from build123d import *

# Parameters (mm, degrees)
SKETCH1_W           = 50
SKETCH1_H           = 45
BOSS_EXTRUDE1_DEPTH = 2
FILLET1_R           = 2
SKETCH3_W           = 3
SKETCH3_H           = 10
SKETCH3_W_2         = 7.936264089
SKETCH3_H_2         = 3
SKETCH3_W_3         = 11
SKETCH3_H_3         = 1.470363465
SKETCH3_H_4         = 1.529636535
SKETCH3_W_4         = 7.991276849
SKETCH3_H_5         = 45
CUT_EXTRUDE1_DEPTH  = 2
SKETCH4_R           = 2
CUT_EXTRUDE2_DEPTH  = 10


with BuildPart() as part:
    # Sketch1 → Boss-Extrude1 (new body)
    with BuildSketch(Plane.XY):
        Polygon((-65, -32.5), (65, -32.5), (65, 32.5), (25, 32.5), (25, -12.5), (-25, -12.5), (-25, 32.5), (-65, 32.5), align=None)
        with Locations((0, 55)):
            Rectangle(SKETCH1_W, SKETCH1_H)
        with Locations((0, 10)):
            Rectangle(SKETCH1_W, SKETCH1_H)
    extrude(amount=BOSS_EXTRUDE1_DEPTH)

    # Fillet1
    fillet1_edges = [part.edges().sort_by_distance(p)[0] for p in [
        (65, 32.5, 1),
        (65, -32.5, 1),
        (-65, -32.5, 1),
        (-65, 32.5, 1),
        (-25, 32.5, 1),
        (-25, 77.5, 1),
        (25, 77.5, 1),
        (25, 32.5, 1),
    ]]
    fillet(fillet1_edges, radius=FILLET1_R)

    # Sketch3 → Cut-Extrude1 (cut)
    with BuildSketch(Plane(origin=(0, 0, 0), x_dir=(-1, 0, 0), z_dir=(0, 0, -1))):
        with Locations((6, 40.5)):
            Rectangle(SKETCH3_W, SKETCH3_H)
        with Locations((-6, 40.5)):
            Rectangle(SKETCH3_W, SKETCH3_H)
        Polygon((-1.5, 34), (0, 34), (0, 47), (-1.5, 47), (-1.5, 45.5), (-1.5, 35.5), align=None)
        Polygon((0, 47), (0, 34), (1.5, 34), (1.5, 35.5), (1.5, 45.5), (1.5, 47), align=None)
        with Locations((-6, 69.5)):
            Rectangle(SKETCH3_W, SKETCH3_H)
        Polygon((-1.5, 63), (0, 63), (0, 76), (-1.5, 76), (-1.5, 74.5), (-1.5, 64.5), align=None)
        Polygon((0, 76), (0, 63), (1.5, 63), (1.5, 64.5), (1.5, 74.5), (1.5, 76), align=None)
        with Locations((6, 69.5)):
            Rectangle(SKETCH3_W, SKETCH3_H)
        with Locations((13.531867956, 60.94842354)):
            Rectangle(SKETCH3_W_2, SKETCH3_H_2)
        with Locations((13.563735911, 55.735181733)):
            Rectangle(SKETCH3_W_3, SKETCH3_H_3)
        with Locations((13.563735911, 54.235181733)):
            Rectangle(SKETCH3_W_3, SKETCH3_H_4)
        with Locations((13.504361575, 48.970363465)):
            Rectangle(SKETCH3_W_4, SKETCH3_H_2)
        with Locations((-13.531867956, 60.94842354)):
            Rectangle(SKETCH3_W_2, SKETCH3_H_2)
        with Locations((-13.563735911, 55.735181733)):
            Rectangle(SKETCH3_W_3, SKETCH3_H_3)
        with Locations((-13.563735911, 54.235181733)):
            Rectangle(SKETCH3_W_3, SKETCH3_H_4)
        with Locations((-13.504361575, 48.970363465)):
            Rectangle(SKETCH3_W_4, SKETCH3_H_2)
        Polygon((-25, 15.428932188), (-17.928932188, 22.5), (-25, 29.571067812), (-32.071067812, 22.5), align=None)
        Polygon((-19, -13), (-19, 13), (-22, 13), (-22, 0), (-22, -13), align=None)
        Polygon((-13, 17), (-13, -17), (-16, -17), (-16, 13), (-16, 17), align=None)
        Polygon((-25, -29.571067812), (-17.928932188, -22.5), (-25, -15.428932188), (-32.071067812, -22.5), align=None)
        with Locations((-54.5, 0)):
            Rectangle(SKETCH3_W, SKETCH3_H_5)
        Polygon((-59, -22.5), (-59, 22.5), (-62, 22.5), (-62, 0), (-62, -22.5), align=None)
        Polygon((25, 29.571067812), (32.071067812, 22.5), (25, 15.428932188), (17.928932188, 22.5), align=None)
        Polygon((22, 0), (22, -13), (19, -13), (19, 13), (22, 13), align=None)
        Polygon((13, 17), (13, -17), (16, -17), (16, 13), (16, 17), align=None)
        Polygon((25, -15.428932188), (32.071067812, -22.5), (25, -29.571067812), (17.928932188, -22.5), align=None)
        Polygon((62, 0), (62, -22.5), (59, -22.5), (59, 22.5), (62, 22.5), align=None)
        with Locations((54.5, 0)):
            Rectangle(SKETCH3_W, SKETCH3_H_5)
    extrude(amount=-CUT_EXTRUDE1_DEPTH, mode=Mode.SUBTRACT)

    # Sketch4 → Cut-Extrude2 (cut)
    with BuildSketch(Plane.XY.offset(2)):
        with Locations((0, -29.5)):
            Circle(SKETCH4_R)
        with Locations((-62, -29.5)):
            Circle(SKETCH4_R)
        with Locations((-13, 36.5)):
            Circle(SKETCH4_R)
        with Locations((13, 36.5)):
            Circle(SKETCH4_R)
        with Locations((62, -29.5)):
            Circle(SKETCH4_R)
        with Locations((22, 74.5)):
            Circle(SKETCH4_R)
        with Locations((-22, 74.5)):
            Circle(SKETCH4_R)
    extrude(amount=-CUT_EXTRUDE2_DEPTH, mode=Mode.SUBTRACT)


solid = part.part
Model file for the job. Use its own axes, mm. A direction names the side the tool comes from. Give positions to 0.01 mm unless a question says otherwise; leave off trailing zeros. Write each loop counter-clockwise with the first axis right and the second up, starting at its lowest first coordinate (ties: lowest second). Pieces come first, ordered by that corner, then holes. Notation, with made-up numbers: M -5,-19 L 38,-19 A10 ccw 38,-2 Z; hole C -34.5,-31 d6. An arc over 180 degrees is marked long. One line per item, written item: value. Start each with the question number.
Q1. 3-axis set-ups, long thin cutter, end or side, ignore diameter. For faces 3 (the flat face through (21.415, -19.014, 0.986)), 4 (the flat face through (-1, 11, 0)): which of +Z, -Z, +X, -X, +Y, -Y reach the whole face in a straight line?
Q2. Saw through at B-B, the plane x = 0. Write the cut outline in (y, z), plus the area to 3 significant figures.
Q3. Drop flat-ended pins along their axis: pin 1 Ø1 at (y, z) = (49, 0.5) entering from +X; pin 2 Ø1 at (y, z) = (61.5, 1.5) entering from -X; pin 3 Ø3 at (x, y) = (22, 74.5) entering from -Z. Give the stop position or say it passes through.
Q4. Saw through at C-C, the plane z = 0.8. State how many separate pieces and enclosed holes the cut face has, plus the area to 3 significant figures.
Q5. Probe probe 1 along Y at (x, z) = (0, 0.9); probe 2 along X at (y, z) = (42.5, 0.55); probe 3 along X at (y, z) = (60, 0.95). List the from-to ranges inside material, lowest first. Write a range as [from, to].
Q6. Saw through at A-A, the plane y = 42.5. Write the cut outline in (x, z).
Q7. Two-plate mould, pull along X, no slides. Class faces 1 (the flat face through (-1, 11, 2)), 2 (the cylindrical face through (-13.434, 34.548, 1.014)): +X half, -X half, draft (parallel to the pull), parting line (faces both ways), or undercut.
Output values:
1. face 3: +Z, -Z
1. face 4: -Z, +X, -X, +Y, -Y
2. outline: M -32.5,0 L -31.5,0 L -31.5,2 L -32.5,2 Z; M -27.5,0 L 34,0 L 34,2 L -27.5,2 Z; M 47,0 L 63,0 L 63,2 L 47,2 Z; M 76,0 L 77.5,0 L 77.5,2 L 76,2 Z
2. area: 160 mm²
3. pin 1: stops at x = 25
3. pin 2: stops at x = -25
3. pin 3: passes through
4. separate pieces: 1
4. enclosed holes: 31
4. area: 8,950 mm²
5. probe 1: y = [-32.5, -31.5], [-27.5, 34], [47, 63], [76, 77.5]
5. probe 2: x = [-25, -7.5], [-4.5, -1.5], [1.5, 4.5], [7.5, 25]
5. probe 3: x = [-25, -17.5], [-9.56, 9.56], [17.5, 25]
6. outline: M -25,0 L -7.5,0 L -7.5,2 L -25,2 Z; M -4.5,0 L -1.5,0 L -1.5,2 L -4.5,2 Z; M 1.5,0 L 4.5,0 L 4.5,2 L 1.5,2 Z; M 7.5,0 L 25,0 L 25,2 L 7.5,2 Z
7. face 1: draft
7. face 2: undercut
